Here's how the part is built. I have some questions about the finished solid (model axes, mm). A direction names the side the tool comes from. Round coordinates to 2 decimals unless told otherwise and drop trailing zeros. Loops run counter-clockwise (first coordinate to the right, second up) from the corner with the lowest first, then second, coordinate; pieces in that order, holes last. Notation, with made-up numbers: (87.5, -35.5) - (121.5, -35.5) arc R15 cw to (121.5, -26.5) - close; hole circle Ø3 at (-30, 47.5). An arc over 180 degrees is marked (long way). Answer as a JSON object with one key per item and string values. Group by question number.
1) If we mould it in two halves opening along X, with no side actions, what happens to faces 1 (the face through (41.402, 53, 2)), 2 (the face through (0, 10, 2)), 3 (the face through (44, 21.167, 2)), 4 (the face through (23.39, 39.74, 2.32))? For each: pulls with the +X half, pulls with the -X half, needs draft (parallel to the pull), parting line crosses it, or undercut.
2) If I drill on line 1 along X through (y, z) = (41.5, 3.1); line 2 along X through (y, z) = (7, 1.2); line 3 along Y through (x, z) = (21.5, 3.9), over which ranges is the centre line in solid material (lowest first)? Write a range as [from, to].
3) I want a section at B-B, the plane x = 24.5. Please give me the cut outline in (y, z).
4) Will these pins go through, and if not, where does the flat tip stop? P1, Ø2.5, axis at x = -2, z = 2, coming from the +Y side; P2, Ø1.4, axis at y = 51, z = 2, coming from the +X side; P3, Ø2.5, axis at y = 12.5, z = 2.5, coming from the -X side.
5) I want a section at C-C, the plane y = 59.5. Please give me the cut outline in (x, z), then the cut area to 3 significant figures.
6) I want a section at A-A, the plane z = 3. Please give me the cut outline in (x, y).
7) Which directions (+Z, -Z, +X, -X, +Y, -Y) give clear straight access to the entire face, cutting with the end or side of a thin tool? Please do faces 5 (the face through (-2, 42.333, 2)), 6 (the face through (15.24, 45, 2)), 7 (the face through (44, 42.333, 2)), 8 (the face through (41.402, 11, 2)).
from build123d import *

# Parameters (mm, degrees)
BOSS_EXTRUDE1_DEPTH = 4.699
SKETCH2_R           = 3.175
CUT_EXTRUDE1_DEPTH  = 79.610640514
CAVITY1_OUTLINE_R   = 3.175
CAVITY1_DEPTH       = 4.699


# Read off the part's stored shape, not the designer's step: Cavity1
with BuildPart() as part:
    # Sketch1 → Boss-Extrude1 (new body)
    with BuildSketch(Plane.XY):
        Polygon((0, 42.333333333), (0, 63.5), (41.402, 63.5), (41.402, 42.333333333), (46.101, 42.333333333), (46.101, 21.166666667), (41.402, 21.166666667), (41.402, 0), (0, 0), (0, 21.166666667), (-4.699, 21.166666667), (-4.699, 42.333333333), align=None)
    extrude(amount=BOSS_EXTRUDE1_DEPTH)

    # Sketch2 → Cut-Extrude1 (cut, through all)
    with BuildSketch(Plane(origin=(0, 0, 0), x_dir=(-1, 0, 0), z_dir=(0, 0, -1))):
        with Locations((-20.701, 44.45)):
            Circle(SKETCH2_R)
    extrude(amount=-CUT_EXTRUDE1_DEPTH, mode=Mode.SUBTRACT)

    # Cavity1 outline → Cavity1 (cut)
    with BuildSketch(Plane.XY):
        Polygon((15.24, 41.34127054), (20.701, 38.18836072), (26.162, 41.34127054), (26.162, 47.64709018), (20.701, 50.8), (15.24, 47.64709018), align=None)
        with Locations((20.701, 44.45)):
            Circle(CAVITY1_OUTLINE_R, mode=Mode.SUBTRACT)
    extrude(amount=CAVITY1_DEPTH, mode=Mode.SUBTRACT)


solid = part.part
Outcome:
{
 "1": {"face 1": "pulls with the +X half", "face 2": "pulls with the -X half", "face 3": "needs draft", "face 4": "undercut"},
 "2": {"line 1": "[-4.7, 15.24], [26.16, 46.1]", "line 2": "[0, 41.4]", "line 3": "[0, 38.65], [50.34, 63.5]"},
 "3": {"outline": "(0, 0) - (40.38, 0) - (40.38, 4.7) - (0, 4.7) - close; (48.61, 0) - (63.5, 0) - (63.5, 4.7) - (48.61, 4.7) - close"},
 "4": {"P1": "y = 42.33", "P2": "x = 41.4", "P3": "x = 0"},
 "5": {"outline": "(0, 0) - (41.4, 0) - (41.4, 4.7) - (0, 4.7) - close", "area": "195 mm^2"},
 "6": {"outline": "(-4.7, 21.17) - (0, 21.17) - (0, 0) - (41.4, 0) - (41.4, 21.17) - (46.1, 21.17) - (46.1, 42.33) - (41.4, 42.33) - (41.4, 63.5) - (0, 63.5) - (0, 42.33) - (-4.7, 42.33) - close; hole (15.24, 41.34) - (20.7, 38.19) - (26.16, 41.34) - (26.16, 47.65) - (20.7, 50.8) - (15.24, 47.65) - close"},
 "7": {"face 5": "+Z, -Z, -X, +Y", "face 6": "+Z, -Z", "face 7": "+Z, -Z, +X, +Y", "face 8": "+Z, -Z, +X, -Y"}
}
